```python
from build123d import *

# Parameters (mm, degrees)
SKETCH_201_R    = 35
EXTRUDE_1_DEPTH = 10
SKETCH_7_R      = 25
EXTRUDE_2_DEPTH = 10
SKETCH_8_R      = 25
EXTRUDE_3_DEPTH = 10
EXTRUDE_4_DEPTH = 10
EXTRUDE_8_DEPTH = 10


with BuildPart() as part:
    # Sketch 201 → Extrude 1 (new body)
    with BuildSketch(Plane(origin=(0, 0, 0), x_dir=(1, 0, 0), z_dir=(0, 1, 0))):
        Circle(SKETCH_201_R)
    extrude(amount=EXTRUDE_1_DEPTH)



with BuildPart() as body_2:
    # Sketch 7 → Extrude 2 (new body)
    with BuildSketch(Plane(origin=(0, 0, 0), x_dir=(1, 0, 0), z_dir=(0, 1, 0))):
        with Locations((-70, -45)):
            Circle(SKETCH_7_R)
    extrude(amount=EXTRUDE_2_DEPTH)


with BuildPart() as body_3:
    # Sketch 8 → Extrude 3 (new body)
    with BuildSketch(Plane(origin=(0, 0, 0), x_dir=(1, 0, 0), z_dir=(0, 1, 0))):
        with Locations((70, -45)):
            Circle(SKETCH_8_R)
    extrude(amount=EXTRUDE_3_DEPTH)


with BuildPart() as body_4:
    # Sketch 9 → Extrude 4 (new body)
    with BuildSketch(Plane(origin=(0, 0, 0), x_dir=(1, 0, 0), z_dir=(0, 1, 0))):
        with BuildLine():
            Line((-90, -116), (90, -116))
            ThreePointArc((90, -116), (97.071067812, -118.928932188), (100, -126))
            Line((100, -126), (100, -130))
            Line((100, -130), (-100, -130))
            Line((-100, -130), (-100, -126))
            ThreePointArc((-100, -126), (-97.071067812, -118.928932188), (-90, -116))
        make_face()
    extrude(amount=EXTRUDE_4_DEPTH)


with BuildPart() as part_1:
    add(part.part)

    add(body_2.part)  # Extrude 8 merges body 2

    add(body_3.part)  # Extrude 8 merges body 3

    add(body_4.part)  # Extrude 8 merges body 4
    # Sketch 21 → Extrude 8 (add)
    with BuildSketch(Plane(origin=(0, 0, 0), x_dir=(1, 0, 0), z_dir=(0, 1, 0))):
        with BuildLine():
            Line((-71.732050808, -116), (-35.936334118, -116))
            ThreePointArc((-35.936334118, -116), (-42.936334118, -114.124355653), (-48.060689771, -109))
            Line((-48.060689771, -109), (-63.822734475, -81.699337741))
            ThreePointArc((-63.822734475, -81.699337741), (-64.701822863, -73.699180065), (-59.401771741, -67.642384101))
            ThreePointArc((-59.401771741, -67.642384101), (-77.500394191, -68.848356064), (-91.650635095, -57.5))
            Line((-91.650635095, -57.5), (-64.803847577, -104))
            ThreePointArc((-64.803847577, -104), (-64.803847577, -112), (-71.732050808, -116))
        make_face()
        with BuildLine():
            Line((7, -104), (7, -42.98837052))
            ThreePointArc((7, -42.98837052), (8.944833021, -36.439048645), (14.14893617, -32.012616345))
            ThreePointArc((14.14893617, -32.012616345), (0, -35), (-14.14893617, -32.012616345))
            ThreePointArc((-14.14893617, -32.012616345), (-8.944833021, -36.439048645), (-7, -42.98837052))
            Line((-7, -42.98837052), (-7, -104))
            ThreePointArc((-7, -104), (-10.514718626, -112.485281374), (-19, -116))
            Line((-19, -116), (19, -116))
            ThreePointArc((19, -116), (10.514718626, -112.485281374), (7, -104))
        make_face()
        with BuildLine():
            ThreePointArc((48.060689771, -109), (42.936334118, -114.124355653), (35.936334118, -116))
            Line((35.936334118, -116), (71.732050808, -116))
            ThreePointArc((71.732050808, -116), (64.803847577, -112), (64.803847577, -104))
            Line((64.803847577, -104), (91.650635095, -57.5))
            ThreePointArc((91.650635095, -57.5), (77.500394191, -68.848356064), (59.401771741, -67.642384101))
            ThreePointArc((59.401771741, -67.642384101), (64.701822863, -73.699180065), (63.822734475, -81.699337741))
            Line((63.822734475, -81.699337741), (48.060689771, -109))
        make_face()
    extrude(amount=EXTRUDE_8_DEPTH)


solid = part_1.part
```
For this review, take the finished solid that the model builds, in its own axes (mm). A direction names the side the tool comes from. Round coordinates to 2 decimals unless told otherwise and drop trailing zeros. Write each loop counter-clockwise with the first axis right and the second up, starting at its lowest first coordinate (ties: lowest second). Pieces come first, ordered by that corner, then holes. Notation, with made-up numbers: (56.5, 46) -> (100.5, 46) arc R15 ccw to (100.5, 61) -> close; hole circle Ø3 at (-7, -25.75). An arc over 180 degrees is marked (long way). One line per question, with ' | ' between items. Start each with the question number.
1) Wall thickness on line 1 along X through (y, z) = (5.25, 46.5); line 2 along X through (y, z) = (8, 77); line 3 along Z through (x, y) = (-52.5, 8.25): over which ranges is each line inside the solid? List them lowest first.
2) For pin 1 Ø1 at (y, z) = (6, 14.5) entering from +X; pin 2 Ø5 at (x, y) = (81.5, 5) entering from -Z; pin 3 Ø1 at (x, y) = (16.5, 2.5) entering from -Z; pin 4 Ø3 at (x, z) = (-1.5, 79.5) entering from -Y, all flat-tipped, find the tip position at first contact; note any pin that passes through.
3) Add section D-D (x = -23). Write out the cut boundary in (y, z).
4) Mouldability with a two-part tool opening along X and no side actions: class faces 5 (the flat face through (-55.83, 4.93, 95.54)), 6 (the cylindrical face through (-64.746, 4.93, 111.898)), 7 (the flat face through (1, 0, 65)) as +X half, -X half, draft (parallel to the pull), parting line (faces both ways), or undercut.
5) Add section A-A (x = -51). Write out the cut boundary in (y, z), and give its area (3 significant figures).
6) Add section B-B (z = 89.5). Write out the cut boundary in (x, y), and give its area (3 significant figures).
7) Machinability: for faces 1 (the flat face through (1, 10, 65)), 2 (the flat face through (56.05, 4.93, 95.16)), 3 (the flat face through (78.039, 4.93, 81.075)), 4 (the flat face through (-81, 5, 116)), which of the approach directions +Z, -Z, +X, -X, +Y, -Y give a long, thin tool a straight path to every point of the face, cutting with its end or side? Answer none if there is none.
8) Add section C-C (y = 7.5). Write out the cut boundary in (x, z), and give its area (3 significant figures).
Reported:
1) line 1: x = -94.95 to -45.05, -7 to 7, 45.05 to 94.95 | line 2: x = -80.39 to -65.16, -7 to 7, 65.16 to 80.39 | line 3: z = 27.15 to 62.85, 101.31 to 130
2) pin 1: stops at x = 32.08 | pin 2: stops at z = 21.68 | pin 3: stops at z = -31.13 | pin 4: stops at y = 0
3) outline: (0, -26.38) -> (10, -26.38) -> (10, 26.38) -> (0, 26.38) -> close; (0, 116) -> (10, 116) -> (10, 130) -> (0, 130) -> close
4) face 5: undercut | face 6: -X half | face 7: draft
5) outline: (0, 28.75) -> (10, 28.75) -> (10, 61.25) -> (0, 61.25) -> close; (0, 103.91) -> (10, 103.91) -> (10, 130) -> (0, 130) -> close | area: 586 mm²
6) outline: (-73.18, 0) -> (-59.32, 0) -> (-59.32, 10) -> (-73.18, 10) -> close; (-7, 0) -> (7, 0) -> (7, 10) -> (-7, 10) -> close; (59.32, 0) -> (73.18, 0) -> (73.18, 10) -> (59.32, 10) -> close | area: 417 mm²
7) face 1: +Z, -Z, +X, -X, +Y | face 2: +Y, -Y | face 3: +X, +Y, -Y | face 4: -X, +Y, -Y
8) outline: (-100, 126) arc R10 ccw to (-90, 116) -> (-71.73, 116) arc R8 cw to (-64.8, 104) -> (-91.65, 57.5) arc R25 ccw (long way) to (-59.4, 67.64) arc R10 cw to (-63.82, 81.7) -> (-48.06, 109) arc R14 cw to (-35.94, 116) -> (-19, 116) arc R12 cw to (-7, 104) -> (-7, 42.99) arc R12 cw to (-14.15, 32.01) arc R35 ccw (long way) to (14.15, 32.01) arc R12 cw to (7, 42.99) -> (7, 104) arc R12 cw to (19, 116) -> (35.94, 116) arc R14 cw to (48.06, 109) -> (63.82, 81.7) arc R10 cw to (59.4, 67.64) arc R25 ccw (long way) to (91.65, 57.5) -> (64.8, 104) arc R8 cw to (71.73, 116) -> (90, 116) arc R10 ccw to (100, 126) -> (100, 130) -> (-100, 130) -> close | area: 13,300 mm²
